Could you check a few things on this model? Use its own coordinates, in mm. A direction names the side the tool comes from. Coordinates: 2 decimals unless noted, no trailing zeros. Write each loop counter-clockwise with the first axis right and the second up, starting at its lowest first coordinate (ties: lowest second). Pieces come first, ordered by that corner, then holes.
Item 1: Thinking about a two-plate mould opening in X: for faces 1 (the cylindrical face through (7.1, 2.6, 49.4)), 2 (the flat face through (0, 1, 28)), 3 (the flat face through (20.833, 1.5, -0.7)), which applies, +X half, -X half, draft (parallel to the pull), parting line (faces both ways), or undercut?
Item 2: If I drill on probe 1 along X at (y, z) = (1.05, 52); probe 2 along Y at (x, z) = (17.5, -1.5); probe 3 along Z at (x, y) = (22, 0.8), over which ranges is the centre line in solid material (lowest first)?
Item 3: I want a section at A-A on x = 8. Please give me the cut outline in (y, z).
Item 4: For P1, Ø0.9, axis at x = 6, y = 1.5, coming from the -Z side; P2, Ø0.9, axis at x = 20.5, y = 1.5, coming from the +Z side; P3, Ø0.9, axis at y = 1.5, z = 51.5, coming from the +X side, each with a flat end and sliding along its axis, tell me the tip position at first contact or that it passes through.
Item 5: Which directions (+Z, -Z, +X, -X, +Y, -Y) give clear straight access to the entire face, cutting with the end or side of a thin tool? Please do faces 4 (the flat face through (7, 2.2, 52)), 5 (the flat face through (24, 1, 47.8)), 6 (the flat face through (26, 2, 0.2)).
Item 6: I want a section at B-B on x = 29.5. Please give me the cut outline in (y, z).
from build123d import *

# Parameters (mm, degrees)
EXTRUDE_1_DEPTH     = 3
SKETCH_2_W          = 9.666666666
SKETCH_2_H          = 3
EXTRUDE_2_DEPTH     = 3
FILLET_1_R          = 1.5
SKETCH_3_R          = 0.65
CUT_EXTRUDE_1_DEPTH = 60.824976204
SKETCH_2_3_W        = 10.666666667
SKETCH_2_3_H        = 3
SKETCH_2_3_W_2      = 0.5
CUT_EXTRUDE_2_DEPTH = 0.2
SKETCH_4_R          = 2.6
CUT_EXTRUDE_3_DEPTH = 0.8
SKETCH_5_R          = 0.35
CUT_EXTRUDE_4_DEPTH = 65.567793829


with BuildPart() as part:
    # 草图1 → 凸台-拉伸1 (new body)
    with BuildSketch(Plane(origin=(0, 0, 0), x_dir=(1, 0, 0), z_dir=(0, 1, 0))):
        Polygon((15.9, -47.8), (32, -47.8), (32, 0), (0, 0), (0, -56), (15.9, -56), align=None)
    extrude(amount=EXTRUDE_1_DEPTH)

    # 草图2 → 凸台-拉伸2 (add)
    with BuildSketch(Plane(origin=(0, 0, 0), x_dir=(-1, 0, 0), z_dir=(0, 0, -1))):
        with Locations((-16, 1.5)):
            Rectangle(SKETCH_2_W, SKETCH_2_H)
    extrude(amount=EXTRUDE_2_DEPTH)

    # 圆角1
    fillet_1_edges = [part.edges().sort_by_distance(p)[0] for p in [
        (16, 3, -3),
        (16, 0, -3),
    ]]
    fillet(fillet_1_edges, radius=FILLET_1_R - 0.0001)  # a hair under: the kernel refuses the full size

    # 草图3 → 切除-拉伸1 (cut, through all)
    with BuildSketch(Plane.ZY.offset(-11.166666667)):
        with Locations((-1.5, 1.5)):
            Circle(SKETCH_3_R)
    extrude(amount=-CUT_EXTRUDE_1_DEPTH, mode=Mode.SUBTRACT)

    # 草图2<3> → 切除-拉伸2 (cut)
    with BuildSketch(Plane(origin=(0, 0, 0), x_dir=(-1, 0, 0), z_dir=(0, 0, -1))):
        with Locations((-5.333333334, 1.5)):
            Rectangle(SKETCH_2_3_W, SKETCH_2_3_H)
        with Locations((-10.916666667, 1.5)):
            Rectangle(SKETCH_2_3_W_2, SKETCH_2_3_H)
        with Locations((-21.083333333, 1.5)):
            Rectangle(SKETCH_2_3_W_2, SKETCH_2_3_H)
        with Locations((-26.666666666, 1.5)):
            Rectangle(SKETCH_2_3_W, SKETCH_2_3_H)
    extrude(amount=-CUT_EXTRUDE_2_DEPTH, mode=Mode.SUBTRACT)

    # 草图4 → 切除-拉伸3 (cut)
    with BuildSketch(Plane(origin=(0, 3, 0), x_dir=(1, 0, 0), z_dir=(0, 1, 0))):
        with Locations(Location((7, -52, 0), (0, 0, 270))):
            Circle(SKETCH_4_R)
    extrude(amount=-CUT_EXTRUDE_3_DEPTH, mode=Mode.SUBTRACT)

    # 草图5 → 切除-拉伸4 (cut, through all)
    with BuildSketch(Plane.XZ):
        with Locations(Location((11.9, 52, 0), (0, 0, 270))):
            Circle(SKETCH_5_R)
        with Locations(Location((4, 52, 0), (0, 0, 270))):
            Circle(SKETCH_5_R)
    extrude(amount=-CUT_EXTRUDE_4_DEPTH, mode=Mode.SUBTRACT)


solid = part.part
Response values:
1. face 1: undercut
1. face 2: -X half
1. face 3: +X half
2. probe 1: x = 0 to 3.65, 4.35 to 11.55, 12.25 to 15.9
2. probe 2: y = 0 to 0.85, 2.15 to 3
2. probe 3: z = 0.2 to 47.8
3. outline: (0, 0.2) - (3, 0.2) - (3, 49.6) - (2.2, 49.6) - (2.2, 54.4) - (3, 54.4) - (3, 56) - (0, 56) - close
4. P1: stops at z = 0.2
4. P2: stops at z = 47.8
4. P3: stops at x = 15.9
5. face 4: +Y
5. face 5: +Z, +X, +Y, -Y
5. face 6: -Z, +X, +Y, -Y
6. outline: (0, 0.2) - (3, 0.2) - (3, 47.8) - (0, 47.8) - close
